Autodesk Fusion 360 part; units mm, degrees
sketch "Sketch1" plane through (0, 0, 0) normal (0, 1, 0) x (1, 0, 0)
  line L0 (0, 0) -> (-50, 0)
  line L1 (-50, 0) -> (-50, 70)
  line L2 (-50, 70) -> (0, 70)
  line L3 (0, 70) -> (0, 0)
  line L4 (-50, 0) -> (-48, 0)
  line L5 (-48, 0) -> (-48, 2)
  line L6 (-48, 2) -> (-50, 2)
  line L7 (-50, 2) -> (-50, 0)
  circle A0 centre (-48, 2) radius 2
  circle A1 centre (-48, 68) radius 2
  circle A2 centre (-2, 68) radius 2
  circle A3 centre (-2, 2) radius 2
  circle A4 centre (-25, 2) radius 2
  circle A5 centre (-25, 68) radius 2
  circle A6 centre (-48, 35) radius 2
  circle A7 centre (-2, 35) radius 2
  line L8 (-23, 68) -> (-23, 70)
  line L9 (-27, 68) -> (-27, 70)
  line L10 (-48, 37) -> (-50, 37)
  line L11 (-48, 33) -> (-50, 33)
  line L12 (-2, 37) -> (0, 37)
  line L13 (-2, 33) -> (0, 33)
  line L14 (-27, 2) -> (-27, 0)
  line L15 (-23, 2) -> (-23, 0)
  line L16 (-4, 2) -> (-4, 0)
  line L17 (-2, 4) -> (0, 4)
  line L18 (-46, 2) -> (-46, 0)
  line L19 (-48, 4) -> (-50, 4)
  line L20 (-48, 66) -> (-50, 66)
  line L21 (-46, 68) -> (-46, 70)
  line L22 (-4, 68) -> (-4, 70)
  line L23 (-2, 66) -> (0, 66)
  line L24 (-23, 70) -> (-27, 70)
  line L25 (-27, 0) -> (-23, 0)
  line L26 (-29, 85) -> (-29, 70)
  line L27 (-21, 87.5) -> (-21, 70)
  line L28 (-29, -15) -> (-29, 0)
  line L29 (-21, -15) -> (-21, 0)
  line L30 (-50, 0) -> (-45, 0)
  line L31 (-45, 5) -> (-5, 5)
  line L32 (-5, 5) -> (-5, 65)
  line L33 (-5, 65) -> (-45, 65)
  line L34 (-45, 65) -> (-45, 5)
  circle A8 centre (-43, 7) radius 2
  circle A9 centre (-7, 7) radius 2
  circle A10 centre (-7, 63) radius 2
  circle A11 centre (-43, 63) radius 2
  circle A12 centre (-48, 68) radius 0.75
  circle A13 centre (-43, 63) radius 0.75
  circle A14 centre (-7, 63) radius 0.75
  circle A15 centre (-2, 68) radius 0.75
  circle A16 centre (-7, 7) radius 0.75
  circle A17 centre (-2, 2) radius 0.75
  circle A18 centre (-48, 2) radius 0.75
  circle A19 centre (-43, 7) radius 0.75
  circle A20 centre (-25, -16) radius 5.05
  circle A21 centre (-25, 86) radius 5.05
  line L35 (-40, 60) -> (-10, 60)
  line L36 (-10, 60) -> (-10, 10)
  line L37 (-10, 10) -> (-40, 10)
  line L38 (-40, 10) -> (-40, 60)
  circle A22 centre (-25, 86) radius 7
  circle A23 centre (-25, -16) radius 7
  dimension "d1" = 50
  dimension "d2" = 70
  dimension "d16" = 1.5
  dimension "d17" = 1.5
  dimension "d18" = 1.5
  dimension "d19" = 1.5
  dimension "d20" = 1.5
  dimension "d21" = 1.5
  dimension "d22" = 1.5
  dimension "d23" = 1.5
  dimension "d24" = 10.1
  dimension "d25" = 10.1
  dimension "d33" = 17.5
extrude "Extrude1" add sketch "Sketch1" along normal blind 3 contours L0 A3 L16 | L0 L1 L2 L3 A0 A1 A2 A3 A4 A5 A6 A7 L8 L9 L10 L11 L12 L13 L14 L15 L16 L17 L18 L19 L20 L21 L22 L23 L30 | L0 L25 L28 L29 A23 | A3 | L0 A4 L15 L25 | L28 L29 A20 A23 | L28 L29 A20 A23 | L3 A3 L17 | L0 A4 L14 L25 | A4 | L3 A7 L13 | L3 A7 L12 | A7 | L0 A0 L18 L30 | L5 L6 A0 A18 | L5 L6 A0 A18 | L3 A2 L23 | L5 L6 A18 | L5 L6 A18 | L1 A0 L19 | A2 | L2 A2 L22 | L1 A6 L11 | L1 A6 L10 | A6 | L2 L24 L26 L27 A22 | L2 A5 L8 L24 | L26 L27 A21 A22 | L26 L27 A21 A22 | L1 A1 L20 | L2 A5 L9 L24 | A5 | A1 | L2 A1 L21 | L31 L34 A8 | L31 L32 L33 L34 A8 A9 A10 A11 | A8 | L31 L32 A9 | A9 | L33 L34 A11 | A11 | L32 L33 A10 | A10 | A12 | A13 | A14 | A15 | A16 | A17 | A19
extrude "Extrude2" add sketch "Sketch1" along normal blind 10 contours A3 | A7 | L5 L6 A0 A18 | L5 L6 A0 A18 | A2 | A6 | A1
extrude "Extrude3" add sketch "Sketch1" along normal blind 8 contours A4 | A5 | A8 | A9 | A11 | A10
fillet "Fillet1" radius 2 12 edges at (-29, 1.5, -70) (-21, 1.5, -70) (-21, 1.5, 0) (-29, 1.5, 0) (-10, 1.5, -60) (-10, 1.5, -10) (-40, 1.5, -10) (-40, 1.5, -60) (-29, 1.5, 10.2554) (-21, 1.5, 10.2554) (-29, 1.5, -80.2554) (-21, 1.5, -80.2554)
extrude "Extrude4" add sketch "Sketch1" along normal blind 6 contours L28 L29 A20 A23 | L28 L29 A20 A23 | L26 L27 A21 A22 | L26 L27 A21 A22
chamfer "Chamfer1" distance 5 distance2 1 2 edges at (-29.7083, 0, -87.8262) (-29.7083, 0, 14.1738) measured on face at (-19.9751, 2, -86.5028) measured on face at (-19.9751, 2, 15.4972)
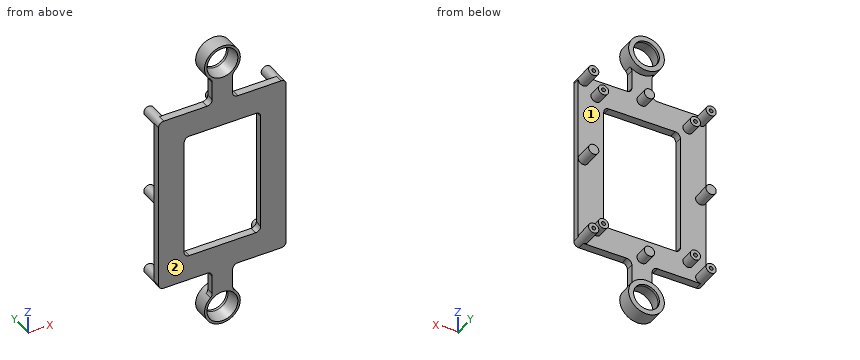
The listing builds one solid part. Answer for the finished solid, in the listing's coordinates (mm). Face numbers are marked on the shaded views. Give positions to 0.01 mm unless a question says otherwise; leave off trailing zeros. Write each loop counter-clockwise with the first axis right and the second up, starting at its lowest first coordinate (ties: lowest second). Pieces come first, ordered by that corner, then holes. Notation, with made-up numbers: (83.25, 54.25) -> (115.25, 54.25) arc R21 ccw to (115.25, 75.25) -> close; hole circle Ø4 at (-14, 87). An arc over 180 degrees is marked (long way). Use a Markdown table: item, result.
(1) Find the intervals of material crossed by probe 1 along Z at (x, y) = (-7, 5.05); probe 2 along Z at (x, y) = (-2, 7.5); probe 3 along Z at (x, y) = (-25, 5.75), in increasing order. Write a range as from..to.
Return value:
| item | result |
|---|---|
| probe 1 | -65..-63.75, -62.25..-61, -9..-7.75, -6.25..-5 |
| probe 2 | -70..-68.75, -67.25..-66, -37..-33, -4..-2.75, -1.25..0 |
| probe 3 | -93..-91.05, -80.95..-79, -70..-66, -4..0, 9..10.95, 21.05..23 |
(2) Section C-C, the plane x = -25 is taken. Give the number of separate pieces and of enclosed holes in the cut face, then the cut area to 3 significant figures.
Return value:
| item | result |
|---|---|
| separate pieces | 4 |
| enclosed holes | 0 |
| area | 191 mm2 |
(3) Section D-D, the plane z = -75.5 is taken. Determine the outline of the cut face in (x, y), then the cut area to 3 significant figures.
Return value:
| item | result |
|---|---|
| outline | (-29, 0) -> (-21, 0) -> (-21, 3) -> (-29, 3) -> close |
| area | 24.0 mm2 |
(4) Determine the mould class of the marked faces 1 and 2 for opening direction Z: released by +Z, released by -Z, zero draft, split by the parting line, or undercut.
Return value:
| item | result |
|---|---|
| face 1 | undercut |
| face 2 | zero draft |
(5) Flat-ended cylindrical pins translate along their axes: P1, Ø0.9, axis at x = -42.5, y = 1, coming from the +Z side; P2, Ø0.9, axis at y = 2, z = 4, coming from the -X side; P3, Ø1.5, axis at x = -21, z = -8, coming from the +Y side; P4, Ø6, axis at x = -25, z = 16, coming from the -Y side. Find the tip coordinate at first contact, or state that the pin passes through.
Return value:
| item | result |
|---|---|
| P1 | z = 0 |
| P2 | x = -29 |
| P3 | y = 3 |
| P4 | through |
(6) Section B-B, the plane z = -53 is taken. Determine the outline of the cut face in (x, y).
Return value:
| item | result |
|---|---|
| outline | (-50, 0) -> (-40, 0) -> (-40, 3) -> (-50, 3) -> close; (-10, 0) -> (0, 0) -> (0, 3) -> (-10, 3) -> close |
(7) Section A-A, the plane x = -14 is taken. Determine the outline of the cut face in (y, z), then the cut area to 3 significant figures.
Return value:
| item | result |
|---|---|
| outline | (0, -70) -> (3, -70) -> (3, -60) -> (0, -60) -> close; (0, -10) -> (3, -10) -> (3, 0) -> (0, 0) -> close |
| area | 60.0 mm2 |
